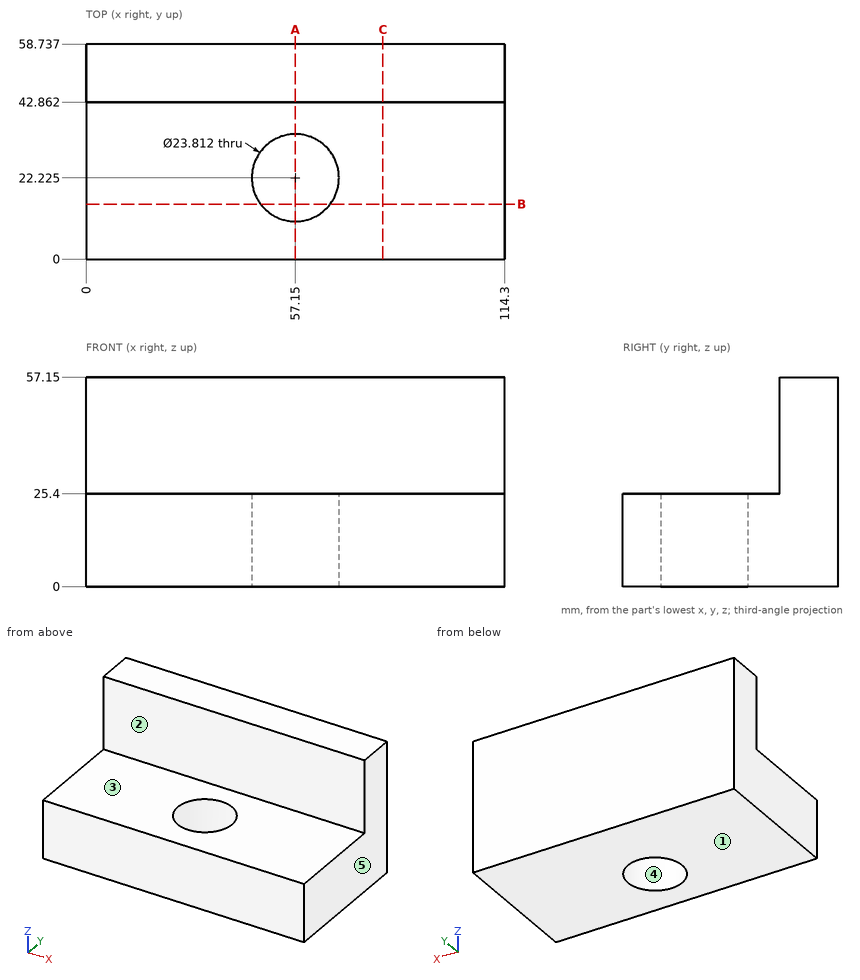
Verification items for this drawing (mm, ordinates from the low corner). A direction names the side the tool comes from. Coordinates: 2 decimals unless noted, no trailing zeros. Loops run counter-clockwise (first coordinate to the right, second up) from the corner with the lowest first, then second, coordinate; pieces in that order, holes last. Notation, with made-up numbers: (0.5, 13) - (45.5, 13) arc R17 cw to (45.5, 30) - close; hole circle Ø3 at (10.5, 75.5). An arc over 180 degrees is marked (long way). Answer as a JSON object with one key per item and string values.
(1) Go/stop test with a flat-tipped pin: pin 1 Ø21.5 at (x, y) = (59, 18.5) entering from +Z. Record where the tip stops, or that it passes through.
Response:
{"pin 1": "stops at z = 25.4"}
(2) Cross-section at C-C, the plane x = 81. Record the boundary of the cut face in (y, z), then the cut area to 3 significant figures.
Response:
{"outline": "(0, 0) - (58.74, 0) - (58.74, 57.15) - (42.86, 57.15) - (42.86, 25.4) - (0, 25.4) - close", "area": "2,000 mm²"}
(3) Scan lines: line 1 along Y through (x, z) = (57, 15); line 2 along Z through (x, y) = (87, 3.5); line 3 along Y through (x, z) = (60, 46). Record each from-to range of solid material in increasing order.
Response:
{"line 1": "y = 0 to 10.32, 34.13 to 58.74", "line 2": "z = 0 to 25.4", "line 3": "y = 42.86 to 58.74"}
(4) Cross-section at B-B, the plane y = 15. Record the boundary of the cut face in (x, z).
Response:
{"outline": "(0, 0) - (47.69, 0) - (47.69, 25.4) - (0, 25.4) - close; (66.61, 0) - (114.3, 0) - (114.3, 25.4) - (66.61, 25.4) - close"}
(5) Cross-section at A-A, the plane x = 57.15. Record the boundary of the cut face in (y, z).
Response:
{"outline": "(0, 0) - (10.32, 0) - (10.32, 25.4) - (0, 25.4) - close; (34.13, 0) - (58.74, 0) - (58.74, 57.15) - (42.86, 57.15) - (42.86, 25.4) - (34.13, 25.4) - close"}
(6) Mould release check, pull along X, two halves, no side actions. Record for the marked faces 3, 4 and 5: pulls with the +X half, pulls with the -X half, needs draft (parallel to the pull), parting line crosses it, or undercut.
Response:
{"face 3": "needs draft", "face 4": "undercut", "face 5": "pulls with the +X half"}
(7) Access from +Z, -Z, +X, -X, +Y, -Y to the whole of each face (thin tool, end or side, straight path). Record for the marked faces 1 and 2.
Response:
{"face 1": "-Z, +X, -X, +Y, -Y", "face 2": "+Z, +X, -X, -Y"}
